Input: dimensioned drawing with shaded views. Units: mm. Origin: part minimum x, y, z. Give positions to 0.01 mm unless a question says otherwise; leave off trailing zeros. Answer in a Markdown table with one row per item. Add a question column.
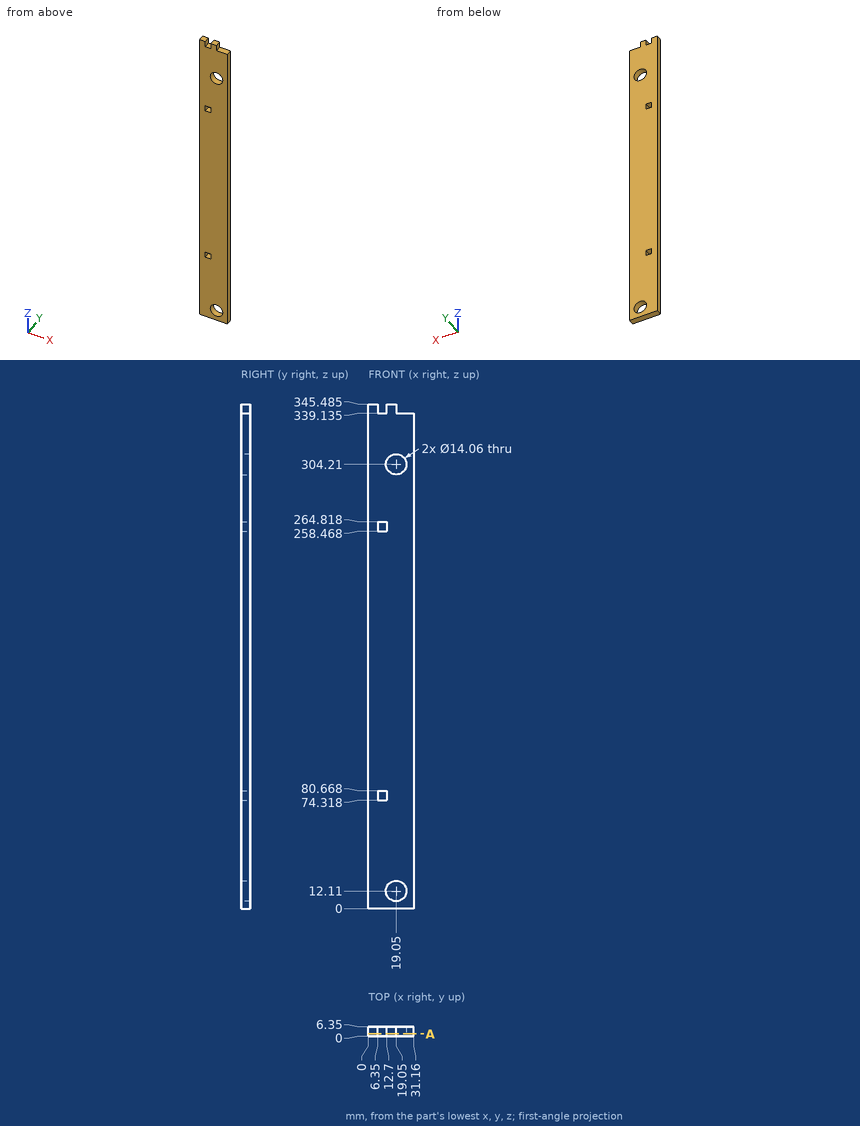
Q1. Contact query for flat-ended pins moving along their axis: pin 1 Ø1.9 at (x, y) = (8.5, 3) entering from +Z (1 decimal); pin 2 Ø4 at (x, z) = (6.5, 165.5) entering from -Y; pin 3 Ø1.9 at (y, z) = (4, 341.5) entering from +X. Output: stop coordinate, or through.
Q2. Line query: probe 1 along X at (y, z) = (1.25, 261); probe 2 along Z at (x, y) = (17, 4) (1 decimal); probe 3 along Z at (x, y) = (21.5, 5.5) (1 decimal). Output: solid intervals per line, ascending. Write a range as from..to.
Q3. Section A-A on y = 1.5. Count the separate pieces of the cut face and the enclosed holes in it, and give its area (3 significant figures).
Checks:
| question | item | result |
|---|---|---|
| 1 | pin 1 | z = 339.1 |
| 1 | pin 2 | y = 0 |
| 1 | pin 3 | x = 19.05 |
| 2 | probe 1 | 0..6.35, 12.7..31.16 |
| 2 | probe 2 | 0..5.4, 18.8..297.5, 310.9..345.5 |
| 2 | probe 3 | 0..5.5, 18.7..297.6, 310.8..339.1 |
| 3 | separate pieces | 1 |
| 3 | enclosed holes | 4 |
| 3 | area | 10,300 mm^2 |
